```python
from build123d import *

# Parameters (mm, degrees)
F0_W     = 88.9
F0_H     = 762
F1_DEPTH = 38.1
F2_W     = 505.46
F2_H     = 38.1
F3_DEPTH = 38.1
F4_W     = 38.1
F4_H     = 762
F5_DEPTH = 38.1
F6_W     = 505.46
F6_H     = 38.1
F7_DEPTH = 38.1


with BuildPart() as f1:
    # F0 (on Front) → F1 (new body)
    with BuildSketch(Plane.XZ):
        Rectangle(F0_W, F0_H)
    extrude(amount=F1_DEPTH)

    # F2 (on Front) → F3 (join)
    with BuildSketch(Plane.XZ):
        with Locations((208.28, 400.05)):
            Rectangle(F2_W, F2_H)
    extrude(amount=F3_DEPTH)

    # F4 (on Front) → F5 (join)
    with BuildSketch(Plane.XZ):
        with Locations((441.96, 0)):
            Rectangle(F4_W, F4_H)
    extrude(amount=F5_DEPTH)

    # F6 (on Front) → F7 (join)
    with BuildSketch(Plane.XZ):
        with Locations((208.28, -400.05)):
            Rectangle(F6_W, F6_H)
    extrude(amount=F7_DEPTH)


solid = f1.part
```
The listing builds one solid part. Answer for the finished solid, in the listing's coordinates (mm). A direction names the side the tool comes from. Give positions to 0.01 mm unless a question says otherwise; leave off trailing zeros. Order: outer loops, then holes, each group sorted by start corner. A loop starts at its lowest first (then second) coordinate and runs counter-clockwise, first axis right, second up. Notation, with made-up numbers: (5.5, 64) -> (51.5, 64) arc R23 cw to (51.5, 87) -> close; hole circle Ø5 at (45.25, 24). An arc over 180 degrees is marked (long way). One line per item, written item: value.
1) Find section B-B, the plane z = 307.5. Determine the outline of the cut face in (x, y).
Reported:
outline: (-44.45, -38.1) -> (44.45, -38.1) -> (44.45, 0) -> (-44.45, 0) -> close; (422.91, -38.1) -> (461.01, -38.1) -> (461.01, 0) -> (422.91, 0) -> close
2) Find section C-C, the plane y = -23.5. Determine the outline of the cut face in (x, z), plus the area to 3 significant figures.
Reported:
outline: (-44.45, -419.1) -> (461.01, -419.1) -> (461.01, 419.1) -> (-44.45, 419.1) -> close; hole (44.45, -381) -> (422.91, -381) -> (422.91, 381) -> (44.45, 381) -> close
area: 135,000 mm^2
3) Find the intervals of material crossed by line 1 (X direction, y = -27.5, z = -164.5); line 2 (Z direction, x = 110, y = -26), in increasing order.
Reported:
line 1: x = -44.45 to 44.45, 422.91 to 461.01
line 2: z = -419.1 to -381, 381 to 419.1
4) A tool of negligible diameter and unlimited length cuts with its end or side. For faces 1 (the flat face through (231, -19, 381)), 2 (the flat face through (461.01, -19, -6)), from which of +Z, -Z, +X, -X, +Y, -Y can it reach the whole face along a straight path? Write none if from no direction.
Reported:
face 1: +Y, -Y
face 2: +Z, -Z, +X, +Y, -Y
5) Determine the mould class of faces 3 (the flat face through (205, -19, 419.1)), 4 (the flat face through (205, -19, -419.1)), 5 (the flat face through (39, -38.1, 33)), 6 (the flat face through (231, -19, -381)) for opening direction Z: pulls with the +Z half, pulls with the -Z half, needs draft (parallel to the pull), parting line crosses it, or undercut.
Reported:
face 3: pulls with the +Z half
face 4: pulls with the -Z half
face 5: needs draft
face 6: undercut
6) Find section A-A, the plane x = 96. Determine the outline of the cut face in (y, z).
Reported:
outline: (-38.1, -419.1) -> (0, -419.1) -> (0, -381) -> (-38.1, -381) -> close; (-38.1, 381) -> (0, 381) -> (0, 419.1) -> (-38.1, 419.1) -> close
